```python
from build123d import *

# Parameters (mm, degrees)
SKETCH_1_W          = 170
SKETCH_1_H          = 40
SKETCH_1_W_2        = 3
SKETCH_1_H_2        = 6
EXTRUDE_2_DEPTH     = 6.5
SKETCH_4_R          = 1.6
CUT_EXTRUDE_1_DEPTH = 25
CUT_EXTRUDE_START   = -25
SKETCH_5_R          = 1.6
CUT_EXTRUDE_2_DEPTH = 25


with BuildPart() as part:
    # 草图1 → 凸台-拉伸2 (new body)
    with BuildSketch(Plane(origin=(0, 0, 0), x_dir=(0, 0, -1), z_dir=(1, 0, 0))):
        with Locations((85, 20)):
            Rectangle(SKETCH_1_W, SKETCH_1_H)
        with Locations((6.5, 4.78605941)):
            Rectangle(SKETCH_1_W_2, SKETCH_1_H_2, mode=Mode.SUBTRACT)
        with Locations((6.5, 35.21394059)):
            Rectangle(SKETCH_1_W_2, SKETCH_1_H_2, mode=Mode.SUBTRACT)
        with Locations((163.5, 4.78605941)):
            Rectangle(SKETCH_1_W_2, SKETCH_1_H_2, mode=Mode.SUBTRACT)
        with Locations((163.5, 35.21394059)):
            Rectangle(SKETCH_1_W_2, SKETCH_1_H_2, mode=Mode.SUBTRACT)
    extrude(amount=EXTRUDE_2_DEPTH)

    # 草图4 → 切除-拉伸1 (cut)
    with BuildSketch(Plane.XY):
        with Locations((3.25, 36.9)):
            Circle(SKETCH_4_R)
        with Locations((3.25, 3.1)):
            Circle(SKETCH_4_R)
    extrude(amount=-CUT_EXTRUDE_1_DEPTH, mode=Mode.SUBTRACT)

    # 草图5 → 切除-拉伸2 (cut)
    with BuildSketch(Plane(origin=(0, 0, -170), x_dir=(-1, 0, 0), z_dir=(0, 0, -1)).offset(CUT_EXTRUDE_START)):
        with Locations(Location((-3.25, 36.9, 0), (0, 0, 180))):
            Circle(SKETCH_5_R)
        with Locations(Location((-3.25, 3.1, 0), (0, 0, 180))):
            Circle(SKETCH_5_R)
    extrude(amount=CUT_EXTRUDE_2_DEPTH, mode=Mode.SUBTRACT)


solid = part.part
```
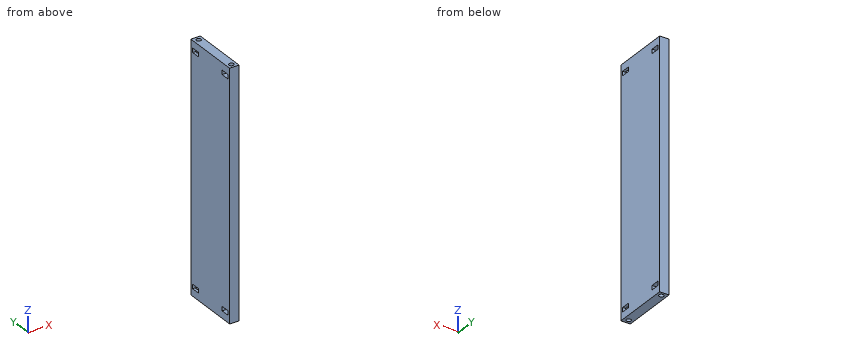
For this review, take the finished solid that the model builds, in its own axes (mm). Give positions to 0.01 mm unless a question says otherwise; leave off trailing zeros. Write each loop counter-clockwise with the first axis right and the second up, starting at its lowest first coordinate (ties: lowest second). Pieces come first, ordered by that corner, then holes.
Item 1: Wall thickness on probe 1 along Y at (x, z) = (3.25, -10.75); probe 2 along Y at (x, z) = (3.25, -164.5); probe 3 along Z at (x, y) = (4.75, 36): over which ranges is each line inside the solid? List them lowest first.
Item 2: Take a section at A-A (z = -151). Give the boundary of the cut face in (x, y), and give its area (3 significant figures).
Item 3: Insertion check: P1, Ø1, axis at x = 3, y = 2.5, coming from the +Z side. The pin has a flat end and moves straight along its axis. Give the tip position at first contact, or say it passes through.
Established:
1. probe 1: y = 0 to 1.5, 4.7 to 35.3, 38.5 to 40
1. probe 2: y = 0 to 1.5, 7.79 to 32.21, 38.5 to 40
1. probe 3: z = -170 to -165, -162 to -8, -5 to 0
2. outline: (0, 0) - (6.5, 0) - (6.5, 40) - (0, 40) - close; hole circle Ø3.2 at (3.25, 3.1); hole circle Ø3.2 at (3.25, 36.9)
2. area: 244 mm2
3. P1: stops at z = -25
